The listing builds one solid part. Answer for the finished solid, in the listing's coordinates (mm). Face numbers are marked on the shaded views. A direction names the side the tool comes from. Give positions to 0.01 mm unless a question says otherwise; leave off trailing zeros. Write each loop counter-clockwise with the first axis right and the second up, starting at its lowest first coordinate (ties: lowest second). Pieces come first, ordered by that corner, then holes. Notation, with made-up numbers: M 52.5,23 L 82.5,23 A28 ccw 82.5,62 Z; hole C 4.5,71 d8. An arc over 180 degrees is marked long. Answer as a JSON object with one key per item and string values.
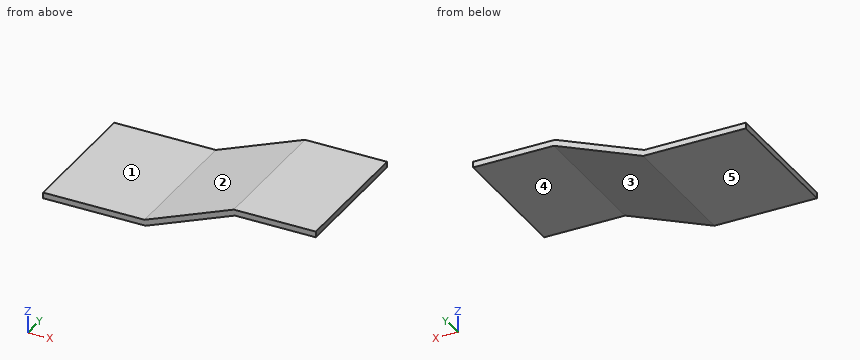
Autodesk Inventor part; units mm, degrees
ref_plane "YZ Plane" through (0, 0, 0) normal (1, 0, 0) x (0, 1, 0)
ref_plane "XZ Plane" through (0, 0, 0) normal (0, 1, 0) x (-1, 0, 0)
ref_plane "XY Plane" through (0, 0, 0) normal (0, 0, 1) x (1, 0, 0)
ref_plane "Work Plane1" through (0, 0, 0) normal (0, 0, 1) x (1, 0, 0)
ref_plane "Work Plane2" through (-64.971, 55, -60) normal (-1, 0, 0) x (0, 0, 1)
sketch "Sketch2" plane through (-64.971, 55, -60) normal (-1, 0, 0) x (0, 0, 1)
  ellipse E0 centre (4.45, -98.8108) end of major axis (-15.5398, -98.8108) minor radius 0.0934
  line L0 (5, -113) -> (60, -113)
  line L1 (60, 3) -> (12.1238, 3)
  line L2 (60, 3) -> (65, 3)
  line L3 (65, 3) -> (65, -113)
  line L4 (65, -113) -> (60, -113)
  line L5 (60, -113) -> (60, 3)
  point P0 (60, -55)
  dimension "d2" = 5
ref_plane "Work Plane3" through (-61.971, -58, -60) normal (0, -1, 0) x (1, 0, 0)
sketch "Sketch3" plane through (-61.971, -58, -60) normal (0, -1, 0) x (1, 0, 0)
  line L0 (-3, 65) -> (-3, 60)
  line L1 (5, 60) -> (84, 60)
  line L2 (160.0104, 90) -> (84, 60)
  line L3 (160.0104, 90) -> (221.6846, 90)
  line L4 (-3, 62.5) -> (84, 62.5)
  line L5 (84, 62.5) -> (160.0104, 92.5)
  spline S0 degree 3 poles (221.6846, 90) (223.5782, 90.3311) (225.4462, 90.6526) (226.8152, 90.8725) (228.4747, 91.1391) (229.032, 91.2163) (229.4035, 91.2679) knots 0 0 0 0 0.710077 0.710077 0.710077 1.570796 1.570796 1.570796 1.570796
  line L6 (160.0104, 92.5) -> (229.4035, 92.5)
  point P0 (61.971, 60)
sweep "Sweep1" add profiles "Sketch2" path "Sketch3" path curves L4 L5 L6 contours L2 L3 L4 L5
properties part number "Lock1"
1. Consider line 1 along Z through (x, y) = (16, 6); line 2 along Z through (x, y) = (143, -44.5). Determine where each line is inside the solid, lowest interval first.
Verdict:
{"line 1": "z = 0 to 5", "line 2": "z = 30 to 35"}
2. For the marked faces 4 and 5, determine the directions among +Z, -Z, +X, -X, +Y, -Y from which every point of the face is accessible in a straight line to the end or side of a thin tool.
Verdict:
{"face 4": "-Z, +X, +Y, -Y", "face 5": "-Z, +X, -X, +Y, -Y"}
3. The mould has two halves that part along X. Classify the marked faces 1, 2 and 3: released by +X, released by -X, zero draft, split by the parting line, or undercut.
Verdict:
{"face 1": "zero draft", "face 2": "released by -X", "face 3": "released by +X"}
4. A cutting plane is placed at C-C, the plane z = 26.5. Give the vertices of the cut face in (x, y), plus the area to 3 significant figures.
Verdict:
{"outline": "M 76.03,-58 L 89.65,-58 L 89.65,58 L 76.03,58 Z", "area": "1,580 mm2"}
5. A cutting plane is placed at B-B, the plane x = -20. Give the vertices of the cut face in (y, z).
Verdict:
{"outline": "M -58,0 L 58,0 L 58,5 L -58,5 Z"}
6. A cutting plane is placed at A-A, the plane y = -44. Give the vertices of the cut face in (x, z).
Verdict:
{"outline": "M -64.97,0 L 22.5,0 L 98.51,30 L 167.43,30 L 167.43,35 L 97.56,35 L 21.55,5 L -64.97,5 Z"}
7. A flat-ended cylindrical pin translates along its axis: pin 1 (4 mm diameter, centred on x = 45.5, y = -32, fed in from -Z). Find the tip coordinate at first contact, or state that the pin passes through.
Verdict:
{"pin 1": "stops at z = 8.29"}
